The listing builds one solid part. Answer for the finished solid, in the listing's coordinates (mm). A direction names the side the tool comes from. Round coordinates to 2 decimals unless told otherwise and drop trailing zeros. Write each loop counter-clockwise with the first axis right and the second up, starting at its lowest first coordinate (ties: lowest second). Pieces come first, ordered by that corner, then holes.
Item 1: Find section A-A on z = 57. Give the vertices of the cut face in (x, y), then the cut area to 3 significant figures.
Item 2: Find the intervals of material crossed by probe 1 along Y at (x, z) = (-1.5, 56); probe 2 along X at (y, z) = (1.5, 24); probe 3 along Z at (x, y) = (-29, 25), in increasing order.
Item 3: For a pull along Y with two mould halves and no side action, classify faces 1 (the face through (-1, 1, -5)), 2 (the face through (-1, 1, 0)), 3 (the face through (25.379, -48.794, 50.314)) as +Y half, -Y half, draft (parallel to the pull), parting line (faces both ways), or undercut.
Item 4: Find section B-B on z = 35.5. Give the vertices of the cut face in (x, y), then the cut area to 3 significant figures.
Item 5: A tool of negligible diameter and unlimited length cuts with its end or side. For faces 4 (the face through (16, -49, 100)), 5 (the face through (-11.056, -49.787, 74.65)), from which of +Z, -Z, +X, -X, +Y, -Y can it reach the whole face along a straight path? Write none if from no direction.
Item 6: Each of these flat-tipped pins is pushed along its axis until it touches: pin 1 (2 mm diameter, centred on x = 16.5, z = 41.5, fed in from +Y); pin 2 (2 mm diameter, centred on x = -22, z = 60.5, fed in from +Y); pin 3 (10 mm diameter, centred on y = 36, z = 10, fed in from -X). Where does it stop, or does it pass through?
```python
from build123d import *

# Parameters (mm, degrees)
F0_R     = 55
F0_R_2   = 51
F0_R_3   = 47
F1_DEPTH = 5
F2_DEPTH = 50
F3_DEPTH = 100
F4_R     = 7


with BuildPart() as f1:
    # F0 (on Top) → F1 (new body)
    with BuildSketch(Plane.XY):
        Circle(F0_R)
        Circle(F0_R_2, mode=Mode.SUBTRACT)
        Circle(F0_R_2)
        Circle(F0_R_3, mode=Mode.SUBTRACT)
        Circle(F0_R_3)
    extrude(amount=-F1_DEPTH)

    # F0 (on Top) → F2 (join)
    with BuildSketch(Plane.XY):
        Circle(F0_R_2)
        Circle(F0_R_3, mode=Mode.SUBTRACT)
    extrude(amount=F2_DEPTH)

    # F0 (on Top) → F3 (join)
    with BuildSketch(Plane.XY):
        Circle(F0_R)
        Circle(F0_R_2, mode=Mode.SUBTRACT)
    extrude(amount=F3_DEPTH)

    # F4
    f4_edges = [f1.edges().sort_by_distance(p)[0] for p in [
        (-55, 0, -5),
    ]]
    fillet(f4_edges, radius=F4_R)


solid = f1.part
```
Check values:
1. outline: circle Ø110 at (0, 0); hole circle Ø102 at (0, 0)
1. area: 1,330 mm2
2. probe 1: y = -54.98 to -50.98, 50.98 to 54.98
2. probe 2: x = -54.98 to -46.98, 46.98 to 54.98
2. probe 3: z = -5 to 0
3. face 1: draft
3. face 2: undercut
3. face 3: parting line
4. outline: circle Ø110 at (0, 0); hole circle Ø94 at (0, 0)
4. area: 2,560 mm2
5. face 4: +Z, +X, -X, +Y, -Y
5. face 5: +Z
6. pin 1: stops at y = 52.77
6. pin 2: stops at y = 50.83
6. pin 3: stops at x = -45.43
